Input: dimensioned drawing with shaded views. Units: mm. Origin: part minimum x, y, z. A direction names the side the tool comes from. Coordinates: 2 decimals unless noted, no trailing zeros. Loops run counter-clockwise (first coordinate to the right, second up) from the corner with the lowest first, then second, coordinate; pieces in that order, holes last.
(1) Line query: L1, parallel to Z at x = 25, y = 3.35; L2, parallel to Z at x = 2.5, y = 25.5; L3, parallel to Y at x = 31.5, z = 15.25. Output: solid intervals per line, ascending.
(2) Section D-D, the plane z = 3. Return loops of the section in (x, y), then the cut area to 3 significant figures.
(3) Section A-A, the plane x = 25. Return loops of the section in (y, z), then the cut area to 3 significant figures.
(4) Mould query, pull axis X, two halves, no side actions, for the marked faces 1, 2, 3 and 4. Classes: released by +X, released by -X, zero draft, split by the parting line, or undercut.
(5) Section C-C, the plane y = 23.5. Return loops of the section in (x, z), then the cut area to 3 significant figures.
(6) Section B-B, the plane x = 17.5. Return loops of the section in (y, z).
(7) Set-up query: the marked faces 5 and 6. Return all of +Z, -Z, +X, -X, +Y, -Y with unobstructed straight access to the full face (end or side cutting, diameter ignored); none if empty.
(8) Contact query for flat-ended pins moving along their axis: P1, Ø10, axis at y = 25.5, z = 16, coming from the +X side; P2, Ø6, axis at y = 17.5, z = 8, coming from the +X side; P3, Ø12, axis at y = 19.5, z = 13, coming from the +X side. Output: stop coordinate, or through.
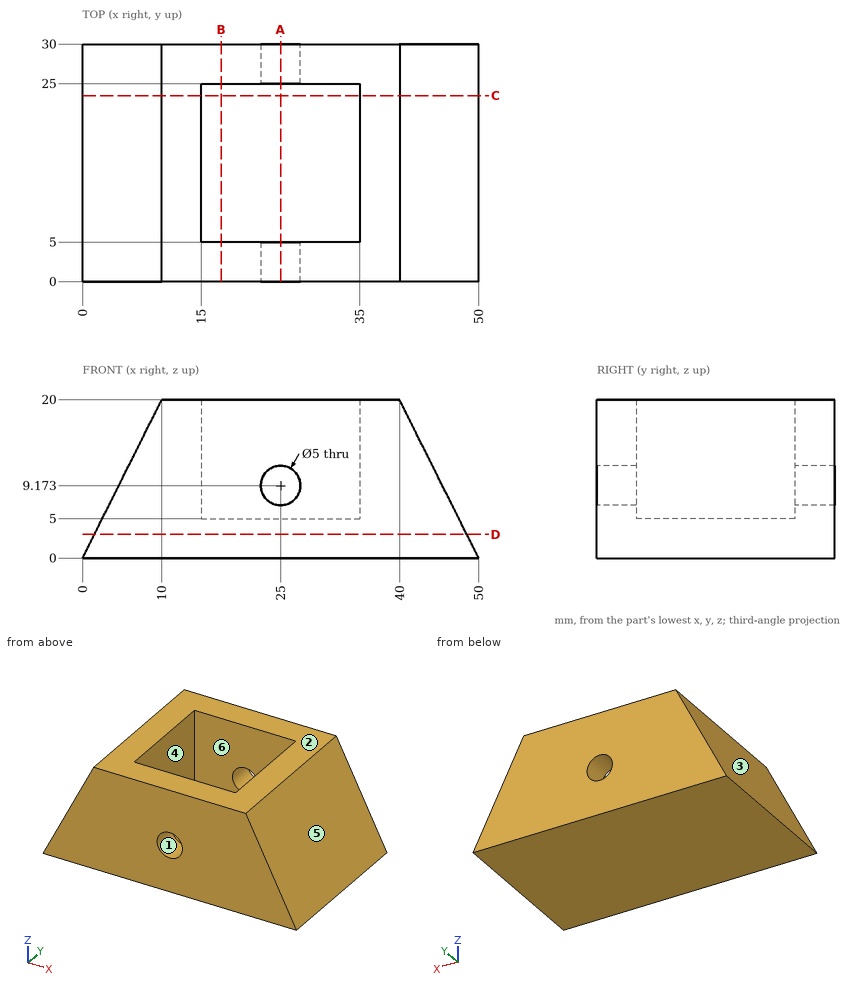
Report:
1. L1: z = 0 to 6.67, 11.67 to 20
1. L2: z = 0 to 5
1. L3: y = 0 to 5, 25 to 30
2. outline: (1.5, 0) - (48.5, 0) - (48.5, 30) - (1.5, 30) - close
2. area: 1,410 mm2
3. outline: (0, 0) - (30, 0) - (30, 6.67) - (25, 6.67) - (25, 5) - (5, 5) - (5, 6.67) - (0, 6.67) - close; (0, 11.67) - (5, 11.67) - (5, 20) - (0, 20) - close; (25, 11.67) - (30, 11.67) - (30, 20) - (25, 20) - close
3. area: 250 mm2
4. face 1: undercut
4. face 2: zero draft
4. face 3: released by -X
4. face 4: undercut
5. outline: (0, 0) - (50, 0) - (40, 20) - (35, 20) - (35, 5) - (15, 5) - (15, 20) - (10, 20) - close
5. area: 500 mm2
6. outline: (0, 0) - (30, 0) - (30, 20) - (25, 20) - (25, 5) - (5, 5) - (5, 20) - (0, 20) - close
7. face 5: +Z, +X, +Y, -Y
7. face 6: +Z
8. P1: stops at x = 44.5
8. P2: stops at x = 47.5
8. P3: stops at x = 46.5
